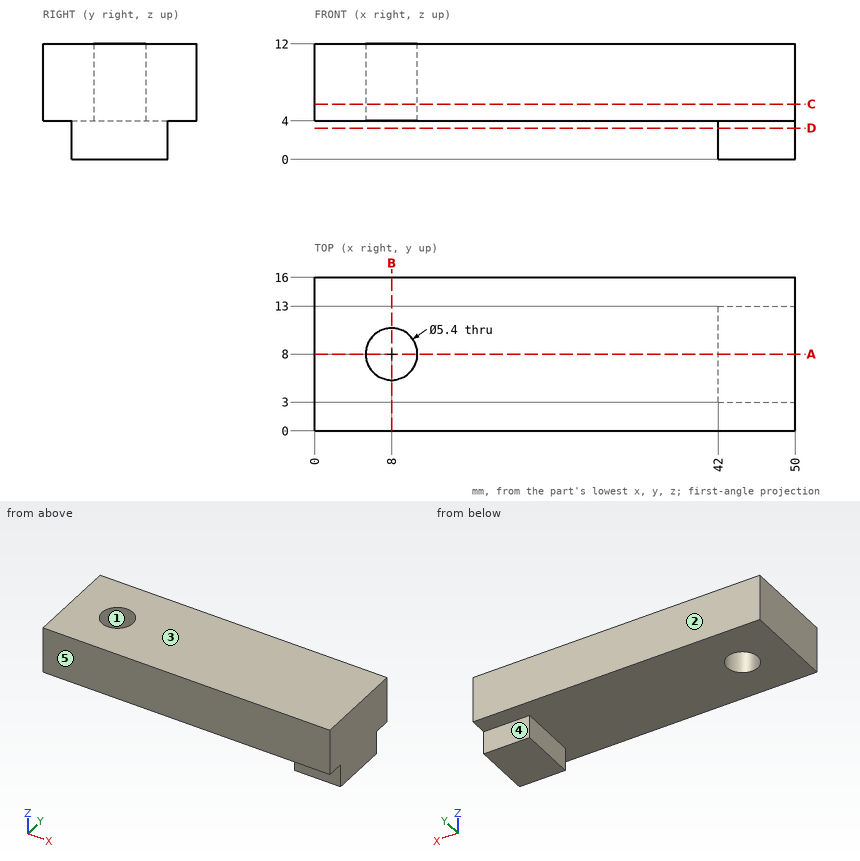
Study the drawing (mm; zero at the part's minimum x, y, z) and answer. A direction names the side the tool comes from. Coordinates: 2 decimals unless noted, no trailing zeros. Write each loop counter-clockwise with the first axis right and the second up, starting at its lowest first coordinate (ties: lowest second). Pieces come first, ordered by that corner, then holes.
Q1. A cutting plane is placed at B-B, the plane x = 8. Give the vertices of the cut face in (y, z), then the cut area to 3 significant figures.
Q2. A cutting plane is placed at D-D, the plane z = 3.25. Give the vertices of the cut face in (x, y), then the cut area to 3 significant figures.
Q3. Determine the mould class of the marked faces 1, 2 and 3 for opening direction Y: released by +Y, released by -Y, zero draft, split by the parting line, or undercut.
Q4. Find the intervals of material crossed by line 1 (Y direction, x = 8, z = 9); line 2 (Z direction, x = 30, y = 3.25); line 3 (X direction, y = 8.5, z = 7), in increasing order.
Q5. Which of the six approach directions +Z, -Z, +X, -X, +Y, -Y give full straight-line access (tool end or side, diameter ignored) to the marked faces 4 and 5?
Q6. A cutting plane is placed at C-C, the plane z = 5.75. Give the vertices of the cut face in (x, y).
Q7. Each of these flat-tipped pins is pushed along its axis until it touches: pin 1 Ø1 at (x, y) = (15.5, 7.5) entering from -Z; pin 2 Ø2 at (x, z) = (47, 1.5) entering from +Y; pin 3 Ø4 at (y, z) = (2.5, 1.5) entering from -X. Where does it stop, or does it pass through?
Q8. A cutting plane is placed at A-A, the plane y = 8. Give the vertices of the cut face in (x, z), then the cut area to 3 significant figures.
Findings below:
1. outline: (0, 4) - (5.3, 4) - (5.3, 12) - (0, 12) - close; (10.7, 4) - (16, 4) - (16, 12) - (10.7, 12) - close
1. area: 84.8 mm2
2. outline: (42, 3) - (50, 3) - (50, 13) - (42, 13) - close
2. area: 80.0 mm2
3. face 1: undercut
3. face 2: released by +Y
3. face 3: zero draft
4. line 1: y = 0 to 5.3, 10.7 to 16
4. line 2: z = 4 to 12
4. line 3: x = 0 to 5.35, 10.65 to 50
5. face 4: -Z, +X, -X, +Y
5. face 5: +Z, -Z, +X, -X, -Y
6. outline: (0, 0) - (50, 0) - (50, 16) - (0, 16) - close; hole circle Ø5.4 at (8, 8)
7. pin 1: stops at z = 4
7. pin 2: stops at y = 13
7. pin 3: stops at x = 42
8. outline: (0, 4) - (5.3, 4) - (5.3, 12) - (0, 12) - close; (10.7, 4) - (42, 4) - (42, 0) - (50, 0) - (50, 12) - (10.7, 12) - close
8. area: 389 mm2
